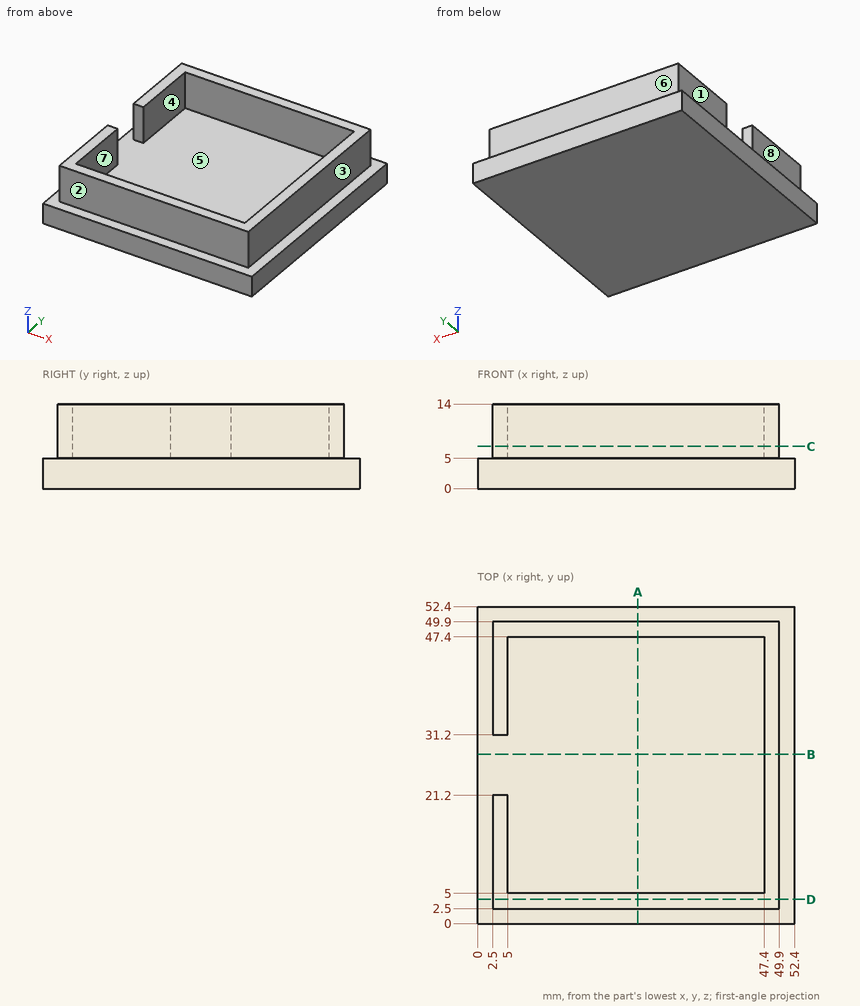
Answer from the drawing. Dimensions are ordinates in mm from the lowest x, y and z of the part. A direction names the side the tool comes from. Give positions to 0.01 mm unless a question says otherwise; leave off trailing zeros. Loops run counter-clockwise (first coordinate to the right, second up) from the corner with the lowest first, then second, coordinate; pieces in that order, holes last. Notation, with made-up numbers: (-3.75, 64) - (47.25, 64) arc R15 ccw to (47.25, 85) - close; hole circle Ø5 at (77, -25). An arc over 180 degrees is marked (long way). Answer as a JSON object with one key per item and string values.
1. For the marked faces 1, 2, 3 and 4, determine the directions among +Z, -Z, +X, -X, +Y, -Y from which every point of the face is accessible in a straight line to the end or side of a thin tool.
Determined:
{"face 1": "+Z, -X, +Y, -Y", "face 2": "+Z, +X, -X, -Y", "face 3": "+Z, +X, +Y, -Y", "face 4": "+Z"}
2. A cutting plane is placed at B-B (y = 28). Write down the section's boundary in (x, z).
Determined:
{"outline": "(0, 0) - (52.4, 0) - (52.4, 5) - (49.9, 5) - (49.9, 14) - (47.4, 14) - (47.4, 5) - (0, 5) - close"}
3. For a pull along Y with two mould halves and no side action, classify the marked faces 5, 6, 7 and 8 as pulls with the +Y half, pulls with the -Y half, needs draft (parallel to the pull), parting line crosses it, or undercut.
Determined:
{"face 5": "undercut", "face 6": "pulls with the +Y half", "face 7": "undercut", "face 8": "needs draft"}
4. A cutting plane is placed at D-D (y = 4). Write down the section's boundary in (x, z), then the cut area to 3 significant figures.
Determined:
{"outline": "(0, 0) - (52.4, 0) - (52.4, 5) - (49.9, 5) - (49.9, 14) - (2.5, 14) - (2.5, 5) - (0, 5) - close", "area": "689 mm²"}
5. Flat-ended cylindrical pins translate along their axes: pin 1 Ø2 at (x, z) = (4, 10) entering from +Y; pin 2 Ø4.5 at (y, z) = (43, 8) entering from -X; pin 3 Ø3 at (y, z) = (41, 11.5) entering from +X. Find the tip coordinate at first contact, or state that the pin passes through.
Determined:
{"pin 1": "y = 49.9", "pin 2": "x = 2.5", "pin 3": "x = 49.9"}
6. A cutting plane is placed at C-C (z = 7). Write down the section's boundary in (x, y).
Determined:
{"outline": "(2.5, 2.5) - (49.9, 2.5) - (49.9, 49.9) - (2.5, 49.9) - (2.5, 31.2) - (5, 31.2) - (5, 47.4) - (47.4, 47.4) - (47.4, 5) - (5, 5) - (5, 21.2) - (2.5, 21.2) - close"}
7. A cutting plane is placed at A-A (x = 26.5). Write down the section's boundary in (y, z).
Determined:
{"outline": "(0, 0) - (52.4, 0) - (52.4, 5) - (49.9, 5) - (49.9, 14) - (47.4, 14) - (47.4, 5) - (5, 5) - (5, 14) - (2.5, 14) - (2.5, 5) - (0, 5) - close"}
8. Find the intervals of material crossed by L1, parallel to X at y = 19.5, z = 5.75; L2, parallel to X at y = 22, z = 10.75, in increasing order. Write a range as [from, to].
Determined:
{"L1": "[2.5, 5], [47.4, 49.9]", "L2": "[47.4, 49.9]"}
